```python
from build123d import *

# Parameters (mm, degrees)
SKETCH1_R           = 1.27
BOSS_EXTRUDE2_DEPTH = 5.08


with BuildPart() as part:
    # Sketch1 → Boss-Extrude2 (new body)
    with BuildSketch(Plane(origin=(0, 0, 0), x_dir=(1, 0, 0), z_dir=(0, 1, 0))):
        with BuildLine():
            Line((-8.953988524, 8.953988524), (-1.208326736, 15.472743004))
            ThreePointArc((-1.208326736, 15.472743004), (-0.025328041, 16.00445947), (1.173542757, 15.50956845))
            Line((1.173542757, 15.50956845), (8.953988524, 8.953988524))
            ThreePointArc((8.953988524, 8.953988524), (0, -12.662852008), (-8.953988524, 8.953988524))
        make_face()
        Circle(SKETCH1_R, mode=Mode.SUBTRACT)
    extrude(amount=BOSS_EXTRUDE2_DEPTH)


solid = part.part
```
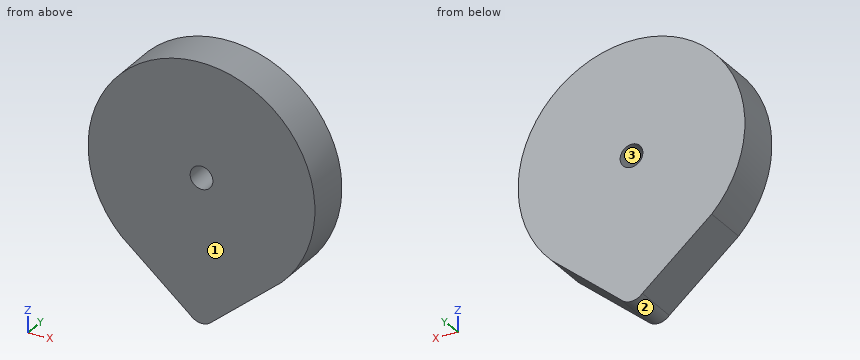
The model under review builds one solid part; all positions refer to its coordinate system, in mm. Face numbers are marked on the shaded views. Round coordinates to 2 decimals unless told otherwise and drop trailing zeros. Loops run counter-clockwise (first coordinate to the right, second up) from the corner with the lowest first, then second, coordinate; pieces in that order, holes last. Notation, with made-up numbers: M 41,65 L 64,65 A36 ccw 64,104 Z; hole C 26.25,2 d9. An arc over 180 degrees is marked long. Write item = value, one per line.
Item 1: Take a section at A-A on z = 0. Write out the cut boundary in (x, y).
Return value:
outline = M -12.66,0 L -1.27,0 L -1.27,5.08 L -12.66,5.08 Z; M 1.27,0 L 12.66,0 L 12.66,5.08 L 1.27,5.08 Z
Item 2: The part is to be moulded in two halves that separate along X. For the marked faces 1, 2 and 3, say which applies: released by +X, released by -X, zero draft, split by the parting line, or undercut.
Return value:
face_1 = zero draft
face_2 = split by the parting line
face_3 = undercut
Item 3: For line 1 (X direction, y = 2.4, z = 0); line 2 (Z direction, x = 0.75, y = 4.85); line 3 (Z direction, x = -6.5, y = 2.7), list the stretches that pass through material, from the lowest coordinate up. Write a range as [from, to].
Return value:
line_1 = [-12.66, -1.27], [1.27, 12.66]
line_2 = [-15.82, -1.02], [1.02, 12.64]
line_3 = [-11.02, 10.87]
Item 4: Take a section at C-C on y = 2.05. Write out the cut boundary in (x, z).
Return value:
outline = M -8.95,-8.95 L -1.21,-15.47 A1.64 ccw 1.17,-15.51 L 8.95,-8.95 A12.66 ccw long Z; hole C 0,0 d2.54
Item 5: Insertion check: P1, Ø2, axis at y = 1.5, z = -3.5, coming from the -X side; P2, Ø1.5, axis at y = 2, z = -10.5, coming from the -X side; P3, Ø2, axis at y = 4.5, z = -4, coming from the -X side; P4, Ø1, axis at x = 7.5, z = 5, coming from the -Y side. Each pin has a flat end and moves straight along its axis. Give the tip position at first contact, or say it passes through.
Return value:
P1 = -12.41
P2 = -8.01
P3 = -12.3
P4 = 0
Item 6: Take a section at D-D on z = -10.5. Write out the cut boundary in (x, y).
Return value:
outline = M -7.12,0 L 7.12,0 L 7.12,5.08 L -7.12,5.08 Z
Item 7: Take a section at B-B on x = 0. Write out the cut boundary in (y, z).
Return value:
outline = M 0,-16 L 5.08,-16 L 5.08,-1.27 L 0,-1.27 Z; M 0,1.27 L 5.08,1.27 L 5.08,12.66 L 0,12.66 Z
